from build123d import *

# Parameters (mm, degrees)
F0_W     = 25
F0_H     = 25
F0_W_2   = 19
F0_H_2   = 19
F1_DEPTH = 120
F2_R     = 1
F3_R     = 3
F5_DEPTH = 25.001
F7_DEPTH = 25.001


with BuildPart() as f1:
    # F0 (on Top) → F1 (new body)
    with BuildSketch(Plane.XY):
        Rectangle(F0_W, F0_H)
        Rectangle(F0_W_2, F0_H_2, mode=Mode.SUBTRACT)
    extrude(amount=F1_DEPTH)

    # F2
    f2_edges = [f1.edges().sort_by_distance(p)[0] for p in [
        (-9.5, -9.5, 60),
        (-9.5, 9.5, 60),
        (9.5, 9.5, 60),
        (9.5, -9.5, 60),
    ]]
    fillet(f2_edges, radius=F2_R)

    # F3
    f3_edges = [f1.edges().sort_by_distance(p)[0] for p in [
        (-12.5, 12.5, 60),
        (-12.5, -12.5, 60),
        (12.5, 12.5, 60),
        (12.5, -12.5, 60),
    ]]
    fillet(f3_edges, radius=F3_R)

    # F4 (on face) → F5 (cut, through all)
    with BuildSketch(Plane.XZ.offset(12.5)):
        Polygon((-9.5, 120), (-9.5, 114.5), (9.5, 95.5), (9.5, 120), align=None)
        Polygon((-9.5, 120), (-15, 120), (-9.5, 114.5), align=None)
        Polygon((9.5, 120), (9.5, 95.5), (15, 90), (15, 120), align=None)
    extrude(amount=-F5_DEPTH, mode=Mode.SUBTRACT)

    # F6 (on face) → F7 (cut, through all)
    with BuildSketch(Plane.YZ.offset(12.5)):
        Polygon((-9.5, 0), (-9.5, 24.5), (-15, 30), (-15, 0), align=None)
        Polygon((9.5, 0), (9.5, 5.5), (-9.5, 24.5), (-9.5, 0), align=None)
        Polygon((9.5, 0), (15, 0), (9.5, 5.5), align=None)
    extrude(amount=-F7_DEPTH, mode=Mode.SUBTRACT)


solid = f1.part
The listing builds one solid part. Answer for the finished solid, in the listing's coordinates (mm). A direction names the side the tool comes from. Coordinates: 2 decimals unless noted, no trailing zeros. Write each loop counter-clockwise with the first axis right and the second up, starting at its lowest first coordinate (ties: lowest second). Pieces come first, ordered by that corner, then holes. Notation, with made-up numbers: M -14,-3 L 26,-3 A22 cw 26,19 Z; hole C 71.5,4.25 d2. An arc over 180 degrees is marked long. Put each result on its own line as item: value. Start each with the question number.
1. A cutting plane is placed at C-C on z = 52. Write down the section's boundary in (x, y), then the cut area to 3 significant figures.
2. Consider line 1 (Y direction, x = -8, z = 62); line 2 (X direction, y = 4.25, z = 101). Determine where each line is inside the solid, lowest interval first. Write a range as from..to.
3. A cutting plane is placed at D-D on y = 11. Write down the section's boundary in (x, z), then the cut area to 3 significant figures.
4. Flat-ended cylindrical pins translate along their axes: P1, Ø1, axis at y = -1.5, z = 102, coming from the +X side; P2, Ø3, axis at x = 3, y = -7, coming from the -Z side; P3, Ø1.5, axis at x = -10, y = -2.5, coming from the +Z side. Find the tip coordinate at first contact, or state that the pin passes through.
5. Which of the six approach directions +Z, -Z, +X, -X, +Y, -Y give full straight-line access (tool end or side, diameter ignored) to faces 1 (the cylindrical face through (-11.64, 11.6, 60.8)), 2 (the flat face through (-9.5, 0, 60))?
6. A cutting plane is placed at A-A on y = -1.75. Write down the section's boundary in (x, z), then the cut area to 4 significant figures.
7. A cutting plane is placed at B-B on x = -0.25. Write down the section's boundary in (y, z), then the cut area to 4 significant figures.
8. For a pull along X with two mould halves and no side action, classify faces 3 (the flat face through (9.5, 0, 50)), 4 (the flat face through (-11, 0, 15)), 5 (the flat face through (12.5, 0, 48)), 6 (the flat face through (0, 9.5, 59)) as pulls with the +X half, pulls with the -X half, needs draft (parallel to the pull), parting line crosses it, or undercut.
Resolved:
1. outline: M -12.5,-9.5 A3 ccw -9.5,-12.5 L 9.5,-12.5 A3 ccw 12.5,-9.5 L 12.5,9.5 A3 ccw 9.5,12.5 L -9.5,12.5 A3 ccw -12.5,9.5 Z; hole M -9.5,-8.5 A1 ccw -8.5,-9.5 L 8.5,-9.5 A1 ccw 9.5,-8.5 L 9.5,8.5 A1 ccw 8.5,9.5 L -8.5,9.5 A1 ccw -9.5,8.5 Z
1. area: 257 mm2
2. line 1: y = -12.5..-9.5, 9.5..12.5
2. line 2: x = -12.5..-9.5
3. outline: M -12.1,4 L 12.1,4 L 12.1,92.9 L -12.1,117.1 Z
3. area: 2,440 mm2
4. P1: stops at x = -9.5
4. P2: passes through
4. P3: stops at z = 115.75
5. face 1: +Z, -Z, -X, +Y
5. face 2: +Z, -Z
6. outline: M -12.5,16.75 L -9.5,16.75 L -9.5,114.5 L -12.5,117.5 Z; M 9.5,16.75 L 12.5,16.75 L 12.5,92.5 L 9.5,95.5 Z
6. area: 529.5 mm2
7. outline: M -12.5,27.5 L -9.5,24.5 L -9.5,105.25 L -12.5,105.25 Z; M 9.5,5.5 L 12.5,2.5 L 12.5,105.25 L 9.5,105.25 Z
7. area: 541.5 mm2
8. face 3: undercut
8. face 4: needs draft
8. face 5: pulls with the +X half
8. face 6: undercut
